```python
from build123d import *

# Parameters (mm, degrees)
BOSS_EXTRUDE3_DEPTH   = 18
SKETCH1_7_W           = 8
SKETCH1_7_H           = 33
BOSS_EXTRUDE4_DEPTH   = 24
BOSS_EXTRUDE4_2_DEPTH = 24
SKETCH1_8_W           = 12
SKETCH1_8_H           = 33
BOSS_EXTRUDE5_DEPTH   = 55
CUT_EXTRUDE1_DEPTH    = 1000
BOSS_EXTRUDE6_DEPTH   = 75
SKETCH1_10_W          = 42
SKETCH1_10_H          = 12
BOSS_EXTRUDE7_DEPTH   = 55
BOSS_EXTRUDE8_DEPTH   = 40


with BuildPart() as part:
    # Sketch1 → Boss-Extrude3 (new body)
    with BuildSketch(Plane(origin=(0, 0, 0), x_dir=(1, 0, 0), z_dir=(0, 1, 0))):
        with BuildLine():
            ThreePointArc((14.170014239, -17.420303066), (-10.829985761, 7.579696934), (-35.829985761, -17.420303066))
            Line((-35.829985761, -17.420303066), (-25.829985761, -17.420303066))
            ThreePointArc((-25.829985761, -17.420303066), (-10.829985761, -2.420303066), (4.170014239, -17.420303066))
            Line((4.170014239, -17.420303066), (14.170014239, -17.420303066))
        make_face()
    extrude(amount=BOSS_EXTRUDE3_DEPTH)



with BuildPart() as body_2:
    # Sketch1_7 → Boss-Extrude4 (new body)
    with BuildSketch(Plane(origin=(0, 0, 0), x_dir=(1, 0, 0), z_dir=(0, 1, 0))):
        with Locations((-44.829985761, -0.920303066)):
            Rectangle(SKETCH1_7_W, SKETCH1_7_H)
    extrude(amount=BOSS_EXTRUDE4_DEPTH)



with BuildPart() as body_3:
    # Sketch1_7 → Boss-Extrude4 2 (new body)
    with BuildSketch(Plane(origin=(0, 0, 0), x_dir=(1, 0, 0), z_dir=(0, 1, 0))):
        with Locations((23.170014239, -0.920303066)):
            Rectangle(SKETCH1_7_W, SKETCH1_7_H)
    extrude(amount=BOSS_EXTRUDE4_2_DEPTH)


with BuildPart() as body_2_1:
    add(body_2.part)

    add(body_3.part)  # Boss-Extrude5 merges body 3
    # Sketch1_8 → Boss-Extrude5 (add)
    with BuildSketch(Plane(origin=(0, 0, 0), x_dir=(1, 0, 0), z_dir=(0, 1, 0))):
        with Locations((-54.829985761, -0.920303066)):
            Rectangle(SKETCH1_8_W, SKETCH1_8_H)
        with Locations((33.170014239, -0.920303066)):
            Rectangle(SKETCH1_8_W, SKETCH1_8_H)
    extrude(amount=BOSS_EXTRUDE5_DEPTH)

    # Sketch2 → Cut-Extrude1 (cut)
    with BuildSketch(Plane.ZY.offset(60.829985761)):
        Polygon((17.420303066, 55), (17.420303066, 24), (-15.579696934, 55), align=None)
    extrude(amount=-CUT_EXTRUDE1_DEPTH, mode=Mode.SUBTRACT)

    # Sketch1_9 → Boss-Extrude6 (add)
    with BuildSketch(Plane(origin=(0, 0, 0), x_dir=(1, 0, 0), z_dir=(0, 1, 0))):
        Polygon((-60.829985761, 27.579696934), (-60.829985761, 15.579696934), (-48.829985761, 15.579696934), (-40.829985761, 15.579696934), (-31.829985761, 15.579696934), (-31.829985761, 27.579696934), align=None)
        Polygon((39.170014239, 27.579696934), (10.170014239, 27.579696934), (10.170014239, 15.579696934), (19.170014239, 15.579696934), (27.170014239, 15.579696934), (39.170014239, 15.579696934), align=None)
    extrude(amount=BOSS_EXTRUDE6_DEPTH)

    # Sketch1_10 → Boss-Extrude7 (add)
    with BuildSketch(Plane(origin=(0, 0, 0), x_dir=(1, 0, 0), z_dir=(0, 1, 0))):
        with Locations((-10.829985761, 21.579696934)):
            Rectangle(SKETCH1_10_W, SKETCH1_10_H)
    extrude(amount=BOSS_EXTRUDE7_DEPTH)


with BuildPart() as part_1:
    add(part.part)

    add(body_2_1.part)  # Boss-Extrude8 merges body 2
    # Sketch1_11 → Boss-Extrude8 (add)
    with BuildSketch(Plane(origin=(0, 0, 0), x_dir=(1, 0, 0), z_dir=(0, 1, 0))):
        with BuildLine():
            Line((-40.829985761, 15.579696934), (-40.829985761, -17.420303066))
            Line((-40.829985761, -17.420303066), (-35.829985761, -17.420303066))
            ThreePointArc((-35.829985761, -17.420303066), (-10.829985761, 7.579696934), (14.170014239, -17.420303066))
            Line((14.170014239, -17.420303066), (19.170014239, -17.420303066))
            Line((19.170014239, -17.420303066), (19.170014239, 15.579696934))
            Line((19.170014239, 15.579696934), (10.170014239, 15.579696934))
            Line((10.170014239, 15.579696934), (-31.829985761, 15.579696934))
            Line((-31.829985761, 15.579696934), (-40.829985761, 15.579696934))
        make_face()
    extrude(amount=BOSS_EXTRUDE8_DEPTH)


solid = part_1.part
```
Verification items for the finished model (mm, model axes). A direction names the side the tool comes from. Round coordinates to 2 decimals unless told otherwise and drop trailing zeros. Order: outer loops, then holes, each group sorted by start corner. A loop starts at its lowest first (then second) coordinate and runs counter-clockwise, first axis right, second up. Notation, with made-up numbers: (-35, -39) - (-18, -39) arc R36 ccw to (-18, -5) - close; hole circle Ø8 at (-39.75, 73). An arc over 180 degrees is marked (long way). Use CSV: the item, a comma, the result in double quotes. Start each with the question number.
1) Access from +Z, -Z, +X, -X, +Y, -Y to the whole of each face (thin tool, end or side, straight path). Record for faces 1 (the flat face through (-11, 40, -10)), 2 (the flat face through (-11, 55, -22)), 3 (the flat face through (-54.914, 39.283, 1.151)), 4 (the cylindrical face through (-11.16, 8.874, 2.424)), 5 (the flat face through (-47, 75, -22)).
2) Go/stop test with flat-tipped pins: P1, Ø6, axis at x = -7.5, z = -19, coming from the +Y side; P2, Ø10, axis at x = -20.5, z = 2, coming from the +Y side; P3, Ø5, axis at x = 27, z = -6, coming from the +Y side. Record where each tip stops, or that it passes through.
3) Section check A-A, the plane y = 68.5. Record the cut outline in (x, z), plus the area to 3 significant figures.
4) Thickness scan on L1, parallel to X at y = 37, z = -8; L2, parallel to X at y = 68, z = -19; L3, parallel to Y at x = 4, z = 13.5. Record the ranges inside material, lowest first.
5) Section check C-C, the plane y = 11. Record the cut outline in (x, z), plus the area to 3 significant figures.
6) Section check D-D, the plane x = -8. Record the cut outline in (y, z).
7) Section check B-B, the plane z = -25. Record the cut outline in (x, y).
Answers:
1,face 1,"+Z, +Y"
1,face 2,"+Z, -Z, +Y"
1,face 3,"+Z, -X, +Y"
1,face 4,"+Z, +Y, -Y"
1,face 5,"+Z, -Z, +X, -X, +Y"
2,P1,"stops at y = 55"
2,P2,"stops at y = 18"
2,P3,"stops at y = 48.34"
3,outline,"(-60.83, -27.58) - (-31.83, -27.58) - (-31.83, -15.58) - (-60.83, -15.58) - close; (10.17, -27.58) - (39.17, -27.58) - (39.17, -15.58) - (10.17, -15.58) - close"
3,area,"696 mm²"
4,L1,"x = -60.83 to -48.83, -40.83 to 19.17, 27.17 to 39.17"
4,L2,"x = -60.83 to -31.83, 10.17 to 39.17"
4,L3,"y = 0 to 18"
5,outline,"(-60.83, -27.58) - (39.17, -27.58) - (39.17, 17.42) - (4.17, 17.42) arc R15 cw to (-25.83, 17.42) - (-60.83, 17.42) - close"
5,area,"4,150 mm²"
6,outline,"(0, -27.58) - (55, -27.58) - (55, -15.58) - (40, -15.58) - (40, -7.42) - (18, -7.42) - (18, 2.69) - (0, 2.69) - close"
7,outline,"(-60.83, 0) - (39.17, 0) - (39.17, 75) - (10.17, 75) - (10.17, 55) - (-31.83, 55) - (-31.83, 75) - (-60.83, 75) - close"
